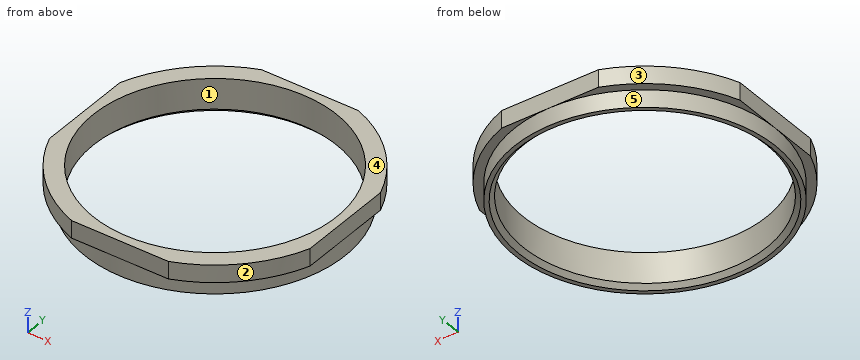
from build123d import *

# Parameters (mm, degrees)
SKETCH001_W   = 50.8
SKETCH001_H   = 50.8
SKETCH001_W_2 = 38.1
SKETCH001_H_2 = 38.1
POCKET_DEPTH  = 5.08
CHAMFER_SIZE  = 0.635


with BuildPart() as part:
    # Sketch → Revolution (revolve)
    with BuildSketch(Plane.XZ):
        Polygon((-17.78, 0), (-20.32, 0), (-20.32, -2.54), (-19.05, -2.54), (-19.05, -5.08), (-17.78, -5.08), align=None)
    revolve(axis=Axis((0, 0, 0), (0, 0, 1)))

    # Sketch001 → Pocket (cut)
    with BuildSketch(Plane.XY):
        Rectangle(SKETCH001_W, SKETCH001_H)
        Rectangle(SKETCH001_W_2, SKETCH001_H_2, mode=Mode.SUBTRACT)
    extrude(amount=-POCKET_DEPTH, mode=Mode.SUBTRACT)

    # Chamfer
    chamfer_edges = [part.edges().sort_by_distance(p)[0] for p in [
        (17.78, 0, -5.08),
    ]]
    chamfer(chamfer_edges, length=CHAMFER_SIZE)


solid = part.part
Verification items for the finished model (mm, model axes). Face numbers are marked on the shaded views. A direction names the side the tool comes from. Give positions to 0.01 mm unless a question says otherwise; leave off trailing zeros. Write each loop counter-clockwise with the first axis right and the second up, starting at its lowest first coordinate (ties: lowest second). Pieces come first, ordered by that corner, then holes.
(1) Access from +Z, -Z, +X, -X, +Y, -Y to the whole of each face (thin tool, end or side, straight path). Record for the marked faces 4 and 5.
(2) Cross-section at A-A (z = -3.1). Enter the section's corners in (x, y), plus the area to 3 significant figures.
(3) Gauge pin test, flat ends, axial feed: pin 1 (8 mm diameter, centred on x = 8.5, y = -11, fed in from -Z); pin 2 (6 mm diameter, centred on x = -12.5, y = -13, fed in from +Z); pin 3 (1.5 mm diameter, centred on y = -12, z = -0.5, fed in from -X); pin 4 (2 mm diameter, centred on y = -8.5, z = -4, fed in from +X). Record the tip position at first contact, or that the pin passes through.
(4) Mould release check, pull along Y, two halves, no side actions. Record for the marked faces 1, 2 and 3: +Y half, -Y half, draft (parallel to the pull), parting line (faces both ways), or undercut.
(5) Material ranges on line 1 (X direction, y = 0, z = -1), recorded low to high.
Worked out:
1. face 4: +Z, +X, -X, +Y, -Y
1. face 5: -Z
2. outline: circle Ø38.1 at (0, 0); hole circle Ø35.56 at (0, 0)
2. area: 147 mm2
3. pin 1: stops at z = -4.57
3. pin 2: stops at z = 0
3. pin 3: stops at x = -16.92
3. pin 4: stops at x = 17.51
4. face 1: undercut
4. face 2: -Y half
4. face 3: +Y half
5. line 1: x = -19.05 to -17.78, 17.78 to 19.05
